Check sheet for the modelled part. Datum: model origin and axes. Units: mm. A direction names the side the tool comes from. Round coordinates to 2 decimals unless told otherwise and drop trailing zeros. Order: outer loops, then holes, each group sorted by start corner. A loop starts at its lowest first (then second) coordinate and runs counter-clockwise, first axis right, second up. Notation, with made-up numbers: (64, 33.25) -> (76, 33.25) arc R21 cw to (76, 71.25) -> close; hole circle Ø11 at (59.5, 72.5). An arc over 180 degrees is marked (long way). Answer in a Markdown table with one row per item.
from build123d import *

# Parameters (mm, degrees)
BOSS_EXTRUDE2_DEPTH = 10
SKETCH2_R           = 2.5
BOSS_EXTRUDE3_DEPTH = 20
SKETCH5_R           = 2.5
BOSS_EXTRUDE4_DEPTH = 30
SKETCH6_R           = 2.5
BOSS_EXTRUDE5_DEPTH = 11.25
FILLET1_R           = 1.25


with BuildPart() as part:
    # Sketch1 → Boss-Extrude2 (new body)
    with BuildSketch(Plane.XY):
        with BuildLine():
            Line((-80, 5), (-30, 5))
            ThreePointArc((-30, 5), (-16.666666667, 10.09288015), (-10.1238402, 22.777777778))
            ThreePointArc((-10.1238402, 22.777777778), (-9.305986892, 24.363389981), (-7.639320225, 25))
            Line((-7.639320225, 25), (5, 25))
            Line((5, 25), (5, 15))
            Line((5, 15), (-5, 15))
            Line((-5, 15), (-5, -15))
            Line((-5, -15), (5, -15))
            Line((5, -15), (5, -25))
            Line((5, -25), (-7.639320225, -25))
            ThreePointArc((-7.639320225, -25), (-9.305986892, -24.363389981), (-10.1238402, -22.777777778))
            ThreePointArc((-10.1238402, -22.777777778), (-16.666666667, -10.09288015), (-30, -5))
            Line((-30, -5), (-80, -5))
            Line((-80, -5), (-80, 5))
        make_face()
    extrude(amount=BOSS_EXTRUDE2_DEPTH)

    # Sketch2 → Boss-Extrude3 (add)
    with BuildSketch(Plane.ZY.offset(80)):
        with Locations((5, 0)):
            Circle(SKETCH2_R)
    extrude(amount=BOSS_EXTRUDE3_DEPTH)

    # Sketch3 → Revolve1 (revolve)
    with BuildSketch(Plane.ZY.offset(100)):
        with BuildLine():
            Line((5, 10), (5, -10))
            ThreePointArc((5, -10), (-5, 0), (5, 10))
        make_face()
    revolve(axis=Axis((-100, 10, 5), (0, -1, 0)))

    # Sketch5 → Boss-Extrude4 (add)
    with BuildSketch(Plane.XZ.offset(-15)):
        with Locations((0, 5)):
            Circle(SKETCH5_R)
    extrude(amount=BOSS_EXTRUDE4_DEPTH)

    # Sketch6 → Boss-Extrude5 (add)
    with BuildSketch(Plane(origin=(0, 25, 0), x_dir=(1, 0, 0), z_dir=(0, 1, 0))):
        with Locations((0, -5)):
            Circle(SKETCH6_R)
    extrude(amount=BOSS_EXTRUDE5_DEPTH)

    # Fillet1
    fillet1_edges = [part.edges().sort_by_distance(p)[0] for p in [
        (-16.666666667, -10.09288015, 10),
        (-55, 5, 0),
        (-16.666666667, 10.09288015, 0),
        (-9.305986892, 24.363389981, 0),
        (-1.319660113, 25, 0),
        (5, 20, 0),
        (0, 15, 0),
        (-5, 0, 0),
        (0, -15, 0),
        (-9.305986892, -24.363389981, 10),
        (5, -20, 0),
        (-1.319660113, -25, 0),
        (-9.305986892, -24.363389981, 0),
        (-16.666666667, -10.09288015, 0),
        (-55, -5, 0),
        (-80, 0, 0),
        (-1.319660113, -25, 10),
        (-80, 5, 5),
        (5, 25, 5),
        (5, 15, 5),
        (5, -15, 5),
        (5, -25, 5),
        (5, -20, 10),
        (-80, -5, 5),
        (0, -15, 10),
        (-5, 0, 10),
        (0, 15, 10),
        (5, 20, 10),
        (-1.319660113, 25, 10),
        (-9.305986892, 24.363389981, 10),
        (-80, 0, 10),
        (-16.666666667, 10.09288015, 10),
        (-55, 5, 10),
        (-55, -5, 10),
    ]]
    fillet(fillet1_edges, radius=FILLET1_R)


solid = part.part
Item 1: Cross-section at C-C (x = -40). Record the boundary of the cut face in (y, z).
Result sheet:
| item | result |
|---|---|
| outline | (-5, 1.25) arc R1.25 ccw to (-3.75, 0) -> (3.75, 0) arc R1.25 ccw to (5, 1.25) -> (5, 8.75) arc R1.25 ccw to (3.75, 10) -> (-3.75, 10) arc R1.25 ccw to (-5, 8.75) -> close |
Item 2: Set-up check for faces 4 (the flat face through (-28, 2, 0)), 5 (the cylindrical face through (-0.33, 0.21, 7.48)), 6 (the flat face through (-55, 5, 5)), 7 (the cylindrical face through (-16.515, -10.23, 4.948)): record each of +Z, -Z, +X, -X, +Y, -Y from which the full face is reachable in a straight line by a thin tool's end or side.
Result sheet:
| item | result |
|---|---|
| face 4 | -Z, +X, +Y, -Y |
| face 5 | none |
| face 6 | +Z, -Z, +Y |
| face 7 | +Z, -Z, -Y |
Item 3: Cross-section at A-A (y = 0). Record the boundary of the cut face in (x, z), and give its area (3 significant figures).
Result sheet:
| item | result |
|---|---|
| outline | (-90.32, 2.5) -> (-80, 2.5) -> (-80, 1.25) arc R1.25 ccw to (-78.75, 0) -> (-6.25, 0) arc R1.25 ccw to (-5, 1.25) -> (-5, 8.75) arc R1.25 ccw to (-6.25, 10) -> (-78.75, 10) arc R1.25 ccw to (-80, 8.75) -> (-80, 7.5) -> (-90.32, 7.5) arc R10 ccw (long way) to start; circle Ø5 at (0, 5) |
| area | 1,130 mm^2 |
Item 4: Depth check by flat-ended pin: P1, Ø6, axis at x = -44.5, z = 4, coming from the +Y side; P2, Ø12, axis at y = -14, z = 10.5, coming from the -X side; P3, Ø8, axis at x = -50.5, y = -8.5, coming from the -Z side; P4, Ø5, axis at x = -93.5, y = 12.5, coming from the +Z side. Enter the tip coordinate at first touch or a pass-through.
Result sheet:
| item | result |
|---|---|
| P1 | stops at y = 5 |
| P2 | stops at x = -104.27 |
| P3 | stops at z = 0.25 |
| P4 | passes through |
Item 5: Cross-section at D-D (y = 31.5). Record the boundary of the cut face in (x, z).
Result sheet:
| item | result |
|---|---|
| outline | circle Ø5 at (0, 5) |
Item 6: Mould release check, pull along X, two halves, no side actions. Record for faces 1 (the flat face through (-2, -25, 5)), 2 (the flat face through (-54, -5, 5)), 3 (the cylindrical face through (-9.29, -24.38, 4.95)): pulls with the +X half, pulls with the -X half, needs draft (parallel to the pull), parting line crosses it, or undercut.
Result sheet:
| item | result |
|---|---|
| face 1 | needs draft |
| face 2 | undercut |
| face 3 | pulls with the -X half |
Item 7: Scan lines: line 1 (Y direction, x = -2.5, z = 6.75); line 2 (Z direction, x = -59, y = -1); line 3 (Y direction, x = -57, z = 4.5). Record each from-to range of solid material in increasing order. Write a range as [from, to].
Result sheet:
| item | result |
|---|---|
| line 1 | y = [-25, -15], [15, 25] |
| line 2 | z = [0, 10] |
| line 3 | y = [-5, 5] |
